Autodesk Inventor part; units mm, degrees
ref_plane "Work Plane2" through (0, 0, 5.5) normal (0, 0, 1) x (1, 0, 0)
ref_plane "Work Plane8" through (0, 0, 0) normal (0.9396926, 0.3420201, 0) x (0, 0, 1)
ref_plane "Work Plane9" through (0, 0, 0) normal (1, 0, 0) x (0, 1, 0)
sketch "Sketch1" plane through (0, 0, 0) normal (0, 0, 1) x (1, 0, 0)
  circle A0 centre (0, 0) radius 5.9792
  dimension "d0" = 11.9585
extrude "Extrusion1" add sketch "Sketch1" along normal blind 11
ref_plane "Work Plane2" through (0, 0, 5.5) normal (0, 0, 1) x (1, 0, 0)
sketch "Sketch2" plane through (0, 0, 0) normal (0, 0, -1) x (-1, 0, 0)
  circle A0 centre (0, 0) radius 5.9792
  circle A1 centre (0, 0) radius 5.15
  dimension "d3" = 10.3
surface extrude "Pitch Diameter" sketch "Sketch2" against normal through all shown no curves A1
ref_plane "Work Plane8" through (0, 0, 0) normal (0.9396926, 0.3420201, 0) x (0, 0, 1)
ref_plane "Work Plane9" through (0, 0, 0) normal (1, 0, 0) x (0, 1, 0)
spur gear teeth "Spur Gear" teeth 9 pitch diameter 11.25 tip diameter 11.9585 root diameter 6.5257 face width 11 start plane through (0, 0, 0) normal (0, 0, -1) x (-1, 0, 0)
equation "\"d0\" = da_da"
equation "\"d1\" = da_b"
equation "\"d3\" = da_dw"
equation "\"d16\" = da_aw"
equation "\"d43\" = da_aw"
equation "\"d46\" = da_aw"
properties part number "Spur Gear2" material "Steel"
Source: CAD feature listing. Evaluate the final solid. Frame: model axes, mm. A direction names the side the tool comes from. Give positions to 0.01 mm unless a question says otherwise; leave off trailing zeros. Order: outer loops, then holes, each group sorted by start corner. A loop starts at its lowest first (then second) coordinate and runs counter-clockwise, first axis right, second up. Notation, with made-up numbers: (59, 4.5) -> (108, 4.5) arc R19 ccw to (108, 20.5) -> close; hole circle Ø3 at (30.25, 12.5). An arc over 180 degrees is marked (long way). Use a Markdown table: item, result.
Q1. Section A-A (y = 4.5). Return the cut outline in (x, z).
A:
| item | result |
|---|---|
| outline | (-3.94, 0) -> (-2.83, 0) -> (-2.83, 11) -> (-3.94, 11) -> close; (-0.85, 0) -> (0.85, 0) -> (0.85, 11) -> (-0.85, 11) -> close; (2.83, 0) -> (3.94, 0) -> (3.94, 11) -> (2.83, 11) -> close |
Q2. Pull-direction query (X, two-part tool) for faces 6 (the face through (2.1, -5.6, 5.4)), 7 (the face through (-0.01, 5.98, 5.42)), 8 (the face through (-2.362, -4.028, 5.423)); classes: +X half, -X half, draft (parallel to the pull), parting line (faces both ways), or undercut.
A:
| item | result |
|---|---|
| face 6 | +X half |
| face 7 | parting line |
| face 8 | undercut |
Q3. First-contact query: P1, Ø4, axis at y = -4.5, z = 6, coming from the -X side; P2, Ø6, axis at y = -1.5, z = 7, coming from the +X side; P3, Ø1.5, axis at x = -4, z = 6, coming from the +Y side; P4, Ø1.5, axis at x = -4.5, z = 4, coming from the +Y side. Flat tips, straight axial feed; report the tip coordinate or a pass-through.
A:
| item | result |
|---|---|
| P1 | x = -5.42 |
| P2 | x = 5.96 |
| P3 | y = 4.9 |
| P4 | y = 4.66 |
Q4. Section D-D (x = 0). Return the cut outline in (y, z).
A:
| item | result |
|---|---|
| outline | (-3.26, 0) -> (5.98, 0) -> (5.98, 11) -> (-3.26, 11) -> close |
Q5. Section B-B (x = -3.75). Return the cut outline in (y, z), and give its area (3 significant figures).
A:
| item | result |
|---|---|
| outline | (-3.11, 0) -> (-1.14, 0) -> (-1.14, 11) -> (-3.11, 11) -> close; (-0.23, 0) -> (1.56, 0) -> (1.56, 11) -> (-0.23, 11) -> close; (3.22, 0) -> (4.66, 0) -> (4.66, 11) -> (3.22, 11) -> close |
| area | 57.1 mm^2 |
Q6. Material intervals for line 1 (Y direction, x = 4, z = 6.5); line 2 (Y direction, x = -3.5, z = 8); line 3 (X direction, y = -4.25, z = 6), sorted ascending. Write a range as [from, to].
A:
| item | result |
|---|---|
| line 1 | [-3.2, -1.29], [-0.19, 1.59], [3.69, 4.44] |
| line 2 | [-3, -1.01], [-0.26, 1.51], [2.83, 4.85] |
| line 3 | [-2.41, -0.61], [0.61, 2.41] |
Q7. Section C-C (y = -4.5). Return the cut outline in (x, z), and give its area (3 significant figures).
A:
| item | result |
|---|---|
| outline | (-2.45, 0) -> (-0.73, 0) -> (-0.73, 11) -> (-2.45, 11) -> close; (0.73, 0) -> (2.45, 0) -> (2.45, 11) -> (0.73, 11) -> close |
| area | 38.0 mm^2 |
Q8. Access query for faces 1 (the face through (0.779, -4.604, 5.423)), 2 (the face through (-4.377, 1.627, 5.423)), 3 (the face through (3.6, 2.98, 5.42)), 4 (the face through (-2.31, 4.06, 5.42)), 5 (the face through (-4.4, -1.57, 5.42)). Directions: +Z, -Z, +X, -X, +Y, -Y. A direction counts if a zero-diameter tool reaches every point of the face in a straight line with its end or side. Return the directions, or none.
A:
| item | result |
|---|---|
| face 1 | +Z, -Z, -Y |
| face 2 | +Z, -Z |
| face 3 | +Z, -Z, +X |
| face 4 | +Z, -Z, +Y |
| face 5 | +Z, -Z, -X |
